The listing builds one solid part. Answer for the finished solid, in the listing's coordinates (mm). A direction names the side the tool comes from. Coordinates: 2 decimals unless noted, no trailing zeros. Loops run counter-clockwise (first coordinate to the right, second up) from the corner with the lowest first, then second, coordinate; pieces in that order, holes last. Notation, with made-up numbers: M 7.5,74 L 58.5,74 A30 cw 58.5,113 Z; hole C 28,70.25 d2. An arc over 180 degrees is marked long. Answer as a JSON object with one key per item and string values. Group by question number.
1. For faces 1 (the face through (26.327, -10.916, 9.86)), 2 (the face through (-4.769, -21.477, -37.989)), determine the directions among +Z, -Z, +X, -X, +Y, -Y from which every point of the face is accessible in a straight line to the end or side of a thin tool.
2. Straight lines are drawn through the part: L1, parallel to Y at x = -1, z = -15; L2, parallel to Z at x = 21, y = -12. For each, find the intervals that lie inside material, in ascending order.
3. Given pin 1 (4 mm diameter, centred on x = -6, z = -6, fed in from -Y); pin 2 (1.5 mm diameter, centred on y = -11.5, z = -15, fed in from -X); pin 3 (3 mm diameter, centred on y = -2.5, z = 7.5, fed in from +X), each flat-ended and moving along its own axis, determine where each tip first touches the part or whether it passes through.
4. A cutting plane is placed at A-A on y = 0. Give the vertices of the cut face in (x, z).
5. A cutting plane is placed at C-C on z = -35.5. Give the vertices of the cut face in (x, y), and give its area (3 significant figures).
from build123d import *

# Parameters (mm, degrees)
SKETCH1_R           = 22
BOSS_EXTRUDE1_DEPTH = 75
SKETCH2_R           = 28.5
BOSS_EXTRUDE2_DEPTH = 20
FILLET1_R           = 2


with BuildPart() as part:
    # Sketch1 → Boss-Extrude1 (new body)
    with BuildSketch(Plane.XY):
        Circle(SKETCH1_R)
    extrude(amount=-BOSS_EXTRUDE1_DEPTH)

    # Sketch2 → Boss-Extrude2 (add)
    with BuildSketch(Plane.XY):
        Circle(SKETCH2_R)
    extrude(amount=BOSS_EXTRUDE2_DEPTH)

    # Fillet1
    fillet1_edges = [part.edges().sort_by_distance(p)[0] for p in [
        (-22, 0, 0),
    ]]
    fillet(fillet1_edges, radius=FILLET1_R)


solid = part.part
From the geometry:
{
 "1": {"face 1": "+Z, -Z", "face 2": "-Z"},
 "2": {"L1": "y = -21.98 to 21.98", "L2": "z = 0 to 20"},
 "3": {"pin 1": "stops at y = -21.63", "pin 2": "stops at x = -19.19", "pin 3": "stops at x = 28.48"},
 "4": {"outline": "M -28.5,0 L -24,0 A2 cw -22,-2 L -22,-75 L 22,-75 L 22,-2 A2 cw 24,0 L 28.5,0 L 28.5,20 L -28.5,20 Z"},
 "5": {"outline": "C 0,0 d44", "area": "1,520 mm²"}
}
